Part model, mm, in its own coordinate system. A direction names the side the tool comes from. Give positions to 0.01 mm unless a question says otherwise; leave off trailing zeros. Loops run counter-clockwise (first coordinate to the right, second up) from the corner with the lowest first, then second, coordinate; pieces in that order, holes last. Notation, with made-up numbers: M -29.5,55.5 L 6.5,55.5 A20 cw 6.5,71.5 Z; hole C 40,41.25 d10. An arc over 180 degrees is marked long. Answer in a Markdown table with one row per item.
from build123d import *

# Parameters (mm, degrees)
BOSS_EXTRUDE1_DEPTH      = 19.05
SKETCH2_R                = 31.75
BOSS_EXTRUDE2_DEPTH      = 19.05
BOSS_EXTRUDE2_DEPTH_BACK = 57.15
CUT_EXTRUDE1_DEPTH       = 197.952392725


with BuildPart() as part:
    # Sketch1 → Boss-Extrude1 (new, symmetric)
    with BuildSketch(Plane(origin=(0, 0, 0), x_dir=(1, 0, 0), z_dir=(0, 1, 0))):
        with BuildLine():
            Line((0, -31.75), (-31.75, -31.75))
            ThreePointArc((-31.75, -31.75), (-85.631536726, -9.431536726), (-107.95, 44.45))
            Line((-107.95, 44.45), (-107.95, 101.6))
            ThreePointArc((-107.95, 101.6), (-76.2, 133.35), (-44.45, 101.6))
            Line((-44.45, 101.6), (-44.45, 57.15))
            ThreePointArc((-44.45, 57.15), (-37.010512242, 39.189487758), (-19.05, 31.75))
            Line((-19.05, 31.75), (0, 31.75))
            Line((0, 31.75), (31.75, 31.75))
            ThreePointArc((31.75, 31.75), (85.631536726, 9.431536726), (107.95, -44.45))
            Line((107.95, -44.45), (107.95, -114.3))
            ThreePointArc((107.95, -114.3), (76.2, -146.05), (44.45, -114.3))
            Line((44.45, -114.3), (44.45, -57.15))
            ThreePointArc((44.45, -57.15), (37.010512242, -39.189487758), (19.05, -31.75))
            Line((19.05, -31.75), (0, -31.75))
        make_face()
    extrude(amount=BOSS_EXTRUDE1_DEPTH, both=True)

    # Sketch2 → Boss-Extrude2 (add, two sides)
    with BuildSketch(Plane(origin=(0, 19.05, 0), x_dir=(1, 0, 0), z_dir=(0, 1, 0))) as boss_extrude2_sk:
        with Locations(Location((-76.2, 101.6, 0), (0, 0, 270))):
            Circle(SKETCH2_R)
        with Locations(Location((76.2, -114.3, 0), (0, 0, 270))):
            Circle(SKETCH2_R)
    extrude(amount=BOSS_EXTRUDE2_DEPTH)
    extrude(boss_extrude2_sk.sketch, amount=-BOSS_EXTRUDE2_DEPTH_BACK)

    # Sketch3 → Cut-Extrude1 (cut, through all)
    with BuildSketch(Plane(origin=(0, 38.1, 0), x_dir=(1, 0, 0), z_dir=(0, 1, 0))):
        with BuildLine():
            Line((-79.375, 125.476), (-73.025, 125.476))
            Line((-73.025, 125.476), (-73.025, 120.383553311))
            ThreePointArc((-73.025, 120.383553311), (-76.2, 82.55), (-79.375, 120.383553311))
            Line((-79.375, 120.383553311), (-79.375, 125.476))
        make_face()
        with BuildLine():
            Line((73.025, -138.176), (79.375, -138.176))
            Line((79.375, -138.176), (79.375, -133.083553311))
            ThreePointArc((79.375, -133.083553311), (76.2, -95.25), (73.025, -133.083553311))
            Line((73.025, -133.083553311), (73.025, -138.176))
        make_face()
    extrude(amount=-CUT_EXTRUDE1_DEPTH, mode=Mode.SUBTRACT)


solid = part.part
(1) Drill centre lines: line 1 along X through (y, z) = (16, 114); line 2 along X through (y, z) = (-4, -101.6); line 3 along Z through (x, y) = (-77, 25). Where is each one in solid material? Low to high.
Recorded:
| item | result |
|---|---|
| line 1 | x = 44.45 to 57.15, 95.25 to 107.95 |
| line 2 | x = -107.95 to -95.25, -57.15 to -44.45 |
| line 3 | z = -133.34 to -125.48, -82.57 to -69.86 |
(2) Saw through at A-A (y = 31.5). Write the cut outline in (x, z) (3 decimals).
Recorded:
| item | result |
|---|---|
| outline | C -76.2,-101.6 d63.5; C 76.2,114.3 d63.5; hole M -79.375,-125.476 L -73.025,-125.476 L -73.025,-120.384 A19.05 ccw long -79.375,-120.384 Z; hole M 73.025,133.084 A19.05 ccw long 79.375,133.084 L 79.375,138.176 L 73.025,138.176 Z |
(3) Pin check, flat tips, straight feed: pin 1 Ø1 at (x, z) = (43.5, -11) entering from -Y; pin 2 Ø6 at (x, y) = (69.5, 30) entering from +Z; pin 3 Ø1.5 at (x, y) = (-83, -12.5) entering from -Z. Stop position of each tip, or through.
Recorded:
| item | result |
|---|---|
| pin 1 | stops at y = -19.05 |
| pin 2 | stops at z = 145.83 |
| pin 3 | stops at z = -132.77 |
(4) Which spindle directions (+Z, -Z, +X, -X, +Y, -Y) get a long thin tool onto all of the face, cutting with end or side? Do faces 1 (the face through (76, 1, 138.176)), 2 (the face through (44.45, 0, 86)), 3 (the face through (-107.95, 0, -73)), 4 (the face through (62.5, -38.1, 128)), 5 (the face through (6, 0, -31.75)). Say none if no direction does.
Recorded:
| item | result |
|---|---|
| face 1 | +Y, -Y |
| face 2 | +Z, -X, +Y, -Y |
| face 3 | +Z, -Z, -X, +Y, -Y |
| face 4 | +Z, -Z, +X, -X, -Y |
| face 5 | -Z, +X, +Y, -Y |
(5) Pull direction X, two halves, no side cores. Call faces 6 (the face through (2, -19.05, 5)), 7 (the face through (-75.407, 0.533, -82.567)), 8 (the face through (-85.036, 0.267, 10.021)), 9 (the face through (-76, 1, -125.476)): +X half, -X half, draft (parallel to the pull), parting line (faces both ways), or undercut.
Recorded:
| item | result |
|---|---|
| face 6 | draft |
| face 7 | undercut |
| face 8 | -X half |
| face 9 | undercut |
(6) Saw through at B-B (y = -1). Write the cut outline in (x, z) (3 decimals), plus the area to 3 significant figures.
Recorded:
| item | result |
|---|---|
| outline | M -107.95,-101.6 A31.75 ccw -44.45,-101.6 L -44.45,-57.15 A25.4 cw -19.05,-31.75 L 31.75,-31.75 A76.2 ccw 107.95,44.45 L 107.95,114.3 A31.75 ccw 44.45,114.3 L 44.45,57.15 A25.4 cw 19.05,31.75 L -31.75,31.75 A76.2 ccw -107.95,-44.45 Z; hole M -79.375,-125.476 L -73.025,-125.476 L -73.025,-120.384 A19.05 ccw long -79.375,-120.384 Z; hole M 73.025,133.084 A19.05 ccw long 79.375,133.084 L 79.375,138.176 L 73.025,138.176 Z |
| area | 22,000 mm^2 |
(7) Saw through at C-C (x = -83.5). Write the cut outline in (y, z), plus the area to 3 significant figures.
Recorded:
| item | result |
|---|---|
| outline | M -38.1,-132.5 L 38.1,-132.5 L 38.1,-119.2 L -38.1,-119.2 Z; M -38.1,-84 L 38.1,-84 L 38.1,-70.7 L 19.05,-70.7 L 19.05,11.48 L -19.05,11.48 L -19.05,-70.7 L -38.1,-70.7 Z |
| area | 5,160 mm^2 |
(8) Saw through at D-D (z = 110). Write the cut outline in (x, y), plus the area to 3 significant figures.
Recorded:
| item | result |
|---|---|
| outline | M 44.45,-19.05 L 44.74,-19.05 L 44.74,-38.1 L 57.64,-38.1 L 57.64,38.1 L 44.74,38.1 L 44.74,19.05 L 44.45,19.05 Z; M 94.76,-38.1 L 107.66,-38.1 L 107.66,-19.05 L 107.95,-19.05 L 107.95,19.05 L 107.66,19.05 L 107.66,38.1 L 94.76,38.1 Z |
| area | 1,990 mm^2 |
